Work out the finished part from the listing and answer in its coordinate system (mm). Give positions to 0.01 mm unless a question says otherwise; leave off trailing zeros. Loops run counter-clockwise (first coordinate to the right, second up) from the corner with the lowest first, then second, coordinate; pieces in that order, holes last. Notation, with made-up numbers: M 53.25,-14.5 L 65.25,-14.5 A18 cw 65.25,20.5 Z; hole C -18.5,-2.75 d4. An arc over 180 degrees is marked long. Write item = value, one per line. Start each with the question number.
1. Section B-B on z = 13.5 is taken. Determine the outline of the cut face in (x, y), plus the area to 3 significant figures.
2. Flat-ended cylindrical pins translate along their axes: pin 1 Ø2 at (x, y) = (19, 1.5) entering from -Z; pin 2 Ø1.9 at (y, z) = (4, -19) entering from -X; pin 3 Ø1.5 at (x, y) = (-32, 4.5) entering from +Z. Find the tip coordinate at first contact, or state that the pin passes through.
3. Section A-A on x = 20 is taken. Determine the outline of the cut face in (y, z), plus the area to 3 significant figures.
4. Consider L1, parallel to X at y = 2, z = -12; L2, parallel to Z at x = -15.5, y = 4.5; L3, parallel to X at y = 2.75, z = -22.5. Determine where each line is inside the solid, lowest interval first. Write a range as [from, to].
5. Section C-C on y = 2.25 is taken. Give the number of separate pieces and of enclosed holes in the cut face, plus the area to 3 significant figures.
```python
from build123d import *

# Parameters (mm, degrees)
SKETCH1_W           = 127
SKETCH1_H           = 114.3
BOSS_EXTRUDE1_DEPTH = 6.35
SKETCH2_W           = 6.35
SKETCH2_H           = 22.86
SKETCH2_W_2         = 25.4
SKETCH2_H_2         = 6.35
CUT_EXTRUDE1_DEPTH  = 7.35
SKETCH3_R           = 1.89865
CUT_EXTRUDE2_DEPTH  = 7.35
SKETCH4_R           = 1.89865
CUT_EXTRUDE3_DEPTH  = 7.35


with BuildPart() as part:
    # Sketch1 → Boss-Extrude1 (new body)
    with BuildSketch(Plane(origin=(0, 0, 0), x_dir=(1, 0, 0), z_dir=(0, 1, 0))):
        Rectangle(SKETCH1_W, SKETCH1_H)
    extrude(amount=BOSS_EXTRUDE1_DEPTH)

    # Sketch2 → Cut-Extrude1 (cut, through all)
    with BuildSketch(Plane(origin=(0, 6.35, 0), x_dir=(1, 0, 0), z_dir=(0, 1, 0))):
        with Locations((-60.325, -22.86)):
            Rectangle(SKETCH2_W, SKETCH2_H)
        with Locations((-60.325, 22.86)):
            Rectangle(SKETCH2_W, SKETCH2_H)
        with Locations((-25.4, 53.975)):
            Rectangle(SKETCH2_W_2, SKETCH2_H_2)
        with Locations((25.4, 53.975)):
            Rectangle(SKETCH2_W_2, SKETCH2_H_2)
        with Locations((60.325, 22.86)):
            Rectangle(SKETCH2_W, SKETCH2_H)
        with Locations((60.325, -22.86)):
            Rectangle(SKETCH2_W, SKETCH2_H)
        with Locations((25.4, -53.975)):
            Rectangle(SKETCH2_W_2, SKETCH2_H_2)
        with Locations((-25.4, -53.975)):
            Rectangle(SKETCH2_W_2, SKETCH2_H_2)
    extrude(amount=-CUT_EXTRUDE1_DEPTH, mode=Mode.SUBTRACT)

    # Sketch3 → Cut-Extrude2 (cut, through all)
    with BuildSketch(Plane(origin=(0, 6.35, 0), x_dir=(1, 0, 0), z_dir=(0, 1, 0))):
        with Locations((-47.076322948, -32.600738686)):
            Circle(SKETCH3_R)
        with Locations((19.598677052, -32.600738686)):
            Circle(SKETCH3_R)
    extrude(amount=-CUT_EXTRUDE2_DEPTH, mode=Mode.SUBTRACT)

    # Sketch4 → Cut-Extrude3 (cut, through all)
    with BuildSketch(Plane.XZ):
        with Locations((-36.916322948, -12.280738686)):
            Circle(SKETCH4_R)
    extrude(amount=-CUT_EXTRUDE3_DEPTH, mode=Mode.SUBTRACT)


solid = part.part
```
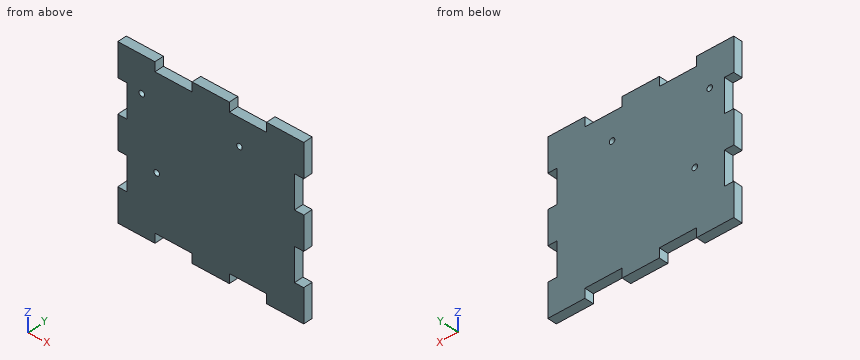
Verdict:
q1.outline = M -57.15,0 L 57.15,0 L 57.15,6.35 L -57.15,6.35 Z
q1.area = 726 mm2
q2.pin_1 = -50.8
q2.pin_2 = -57.15
q2.pin_3 = 50.8
q3.outline = M 0,-50.8 L 6.35,-50.8 L 6.35,30.74 L 0,30.74 Z; M 0,34.46 L 6.35,34.46 L 6.35,50.8 L 0,50.8 Z
q3.area = 622 mm2
q4.L1 = [-57.15, -38.79], [-35.04, 57.15]
q4.L2 = [-50.8, 50.8]
q4.L3 = [-57.15, 57.15]
q5.separate_pieces = 1
q5.enclosed_holes = 3
q5.area = 13,300 mm2
